The model under review builds one solid part; all positions refer to its coordinate system, in mm. Face numbers are marked on the shaded views. A direction names the side the tool comes from. Give positions to 0.01 mm unless a question says otherwise; leave off trailing zeros. Loops run counter-clockwise (first coordinate to the right, second up) from the corner with the lowest first, then second, coordinate; pieces in that order, holes last. Notation, with made-up numbers: M -28.5,33 L -21.5,33 A27 ccw -21.5,52 Z; hole C 16,-28.5 d3. An arc over 180 degrees is marked long. Put each result on its own line as item: value. Start each with the question number.
from build123d import *

# Parameters (mm, degrees)
F0_R     = 22.86
F1_DEPTH = 3.175
F2_W     = 8.89
F2_H     = 3.048
F3_DEPTH = 9.652
F4_R     = 1.5875
F5_DEPTH = 24.385
F6_R     = 0.508
F7_R     = 0.381


with BuildPart() as f1:
    # F0 (on Front) → F1 (new body)
    with BuildSketch(Plane.XZ):
        Circle(F0_R)
    extrude(amount=F1_DEPTH)

    # F2 (on face) → F3 (join)
    with BuildSketch(Plane.XZ.offset(3.175)):
        Rectangle(F2_W, F2_H)
    extrude(amount=F3_DEPTH)

    # F4 (on face) → F5 (cut, through all)
    with BuildSketch(Plane(origin=(0, 0, -1.524), x_dir=(1, 0, 0), z_dir=(0, 0, -1))):
        with Locations((0, 6.35)):
            Circle(F4_R)
    extrude(amount=-F5_DEPTH, mode=Mode.SUBTRACT)

    # F6
    f6_edges = [f1.edges().sort_by_distance(p)[0] for p in [
        (-4.445, -12.827, 0),
        (4.445, -12.827, 0),
        (0, -3.175, -1.524),
        (-4.445, -3.175, 0),
        (4.445, -3.175, 0),
        (0, -3.175, 1.524),
    ]]
    fillet(f6_edges, radius=F6_R)

    # F7
    f7_edges = [f1.edges().sort_by_distance(p)[0] for p in [
        (-22.86, -3.175, 0),
        (-22.86, 0, 0),
    ]]
    fillet(f7_edges, radius=F7_R)


solid = f1.part
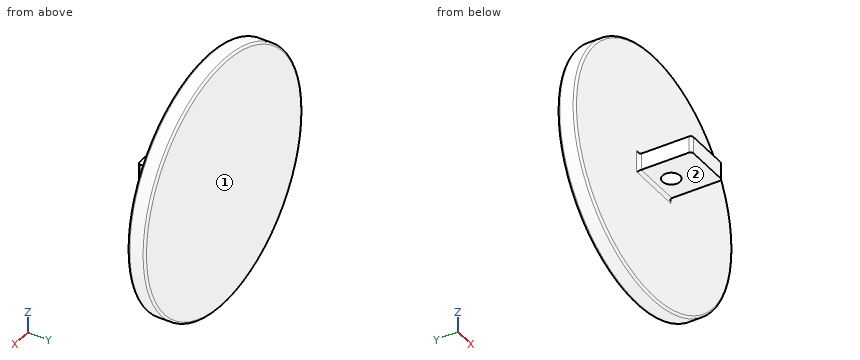
(1) We need section D-D, the plane y = -11.75. Write out the cut boundary in (x, z) (3 decimals).
(2) We need section B-B, the plane y = -6.35. Write out the cut boundary in (x, z) (1 decimal), plus the area to 3 significant figures.
(3) We need section C-C, the plane x = 0. Write out the cut boundary in (y, z) (1 decimal).
(4) To check wall thickness, follow L1, parallel to Y at x = 0, z = 0; L2, parallel to Y at x = -9, z = -16.5 (3 decimals); L3, parallel to Z at x = 1, y = -8.75. State the ranges of each line that lie inside material, in increasing order. Write a range as [from, to].
(5) Insertion check: pin 1 (2 mm diameter, centred on y = -3, z = 7, fed in from -X); pin 2 (1 mm diameter, centred on x = -1.5, y = -10.5, fed in from +Z); pin 3 (2 mm diameter, centred on x = -10.5, z = 17, fed in from -Y) (3 decimals). Each pin has a flat end and moves straight along its axis. Give the tip position at first contact, or say it passes through.
(6) For the marked faces 1 and 2, list the 3-axis set-ups (+Z, -Z, +X, -X, +Y, -Y) from which the entire face can be reached by the end or side of a thin tool; tool diameter is ignored.
Check sheet entries:
1. outline: M -4.445,-1.524 L 4.445,-1.524 L 4.445,1.524 L -4.445,1.524 Z
2. outline: M -4.4,-1.5 L -1.6,-1.5 L -1.6,1.5 L -4.4,1.5 Z; M 1.6,-1.5 L 4.4,-1.5 L 4.4,1.5 L 1.6,1.5 Z
2. area: 17.4 mm²
3. outline: M -12.8,-1.5 L -7.9,-1.5 L -7.9,1.5 L -12.8,1.5 Z; M -4.8,-1.5 L -3.7,-1.5 A0.5 cw -3.2,-2 L -3.2,-22.5 A0.4 ccw -2.8,-22.9 L -0.4,-22.9 A0.4 ccw 0,-22.5 L 0,22.5 A0.4 ccw -0.4,22.9 L -2.8,22.9 A0.4 ccw -3.2,22.5 L -3.2,2 A0.5 cw -3.7,1.5 L -4.8,1.5 Z
4. L1: y = [-12.83, -7.94], [-4.76, 0]
4. L2: y = [-3.175, 0]
4. L3: z = [-1.52, 1.52]
5. pin 1: stops at x = -22.05
5. pin 2: stops at z = 1.52
5. pin 3: stops at y = -3.175
6. face 1: +Z, -Z, +X, -X, +Y
6. face 2: -Z, +X, -X, -Y
